Work out the finished part from the listing and answer in its coordinate system (mm). Give positions to 0.01 mm unless a question says otherwise; leave off trailing zeros. Write each loop counter-clockwise with the first axis right and the second up, starting at its lowest first coordinate (ties: lowest second). Pieces come first, ordered by that corner, then holes.
1) Given pin 1 Ø3 at (y, z) = (236, -1.5) entering from +X; pin 2 Ø5 at (y, z) = (98.5, 7.5) entering from +X; pin 3 Ø8 at (x, z) = (-358, -4) entering from -Y, each flat-ended and moving along its own axis, determine where each tip first touches the part or whether it passes through.
2) Straight lines are drawn through the part: probe 1 along X at (y, z) = (385.5, -10); probe 2 along X at (y, z) = (368, 12); probe 3 along Y at (x, z) = (-140.5, 21). For each, find the intervals that lie inside material, in ascending order.
3) Find section A-A (z = 8.5). Determine the outline of the cut face in (x, y) (1 decimal), plus the area to 3 significant figures.
4) Find section B-B (x = -89). Determine the outline of the cut face in (y, z), plus the area to 3 significant figures.
5) Find section C-C (y = 63). Determine the outline of the cut face in (x, z), plus the area to 3 significant figures.
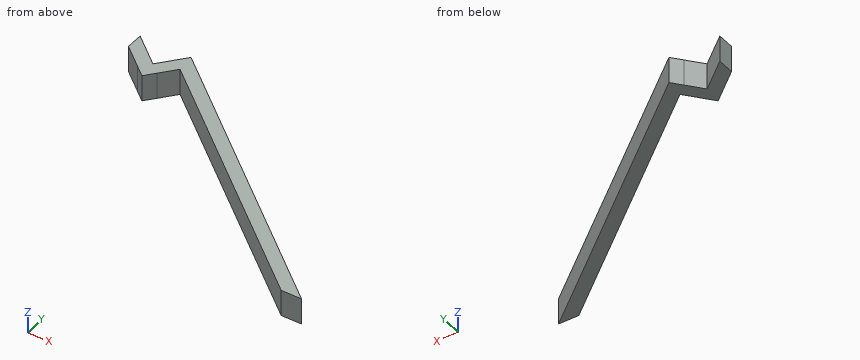
Autodesk Inventor part; units mm, degrees
ref_plane "YZ Plane" through (0, 0, 0) normal (1, 0, 0) x (0, 1, 0)
ref_plane "XZ Plane" through (0, 0, 0) normal (0, 1, 0) x (-1, 0, 0)
ref_plane "XY Plane" through (0, 0, 0) normal (0, 0, 1) x (1, 0, 0)
sketch "Sketch1" plane through (0, 0, 0) normal (0, 0, 1) x (1, 0, 0)
  line L0 (0, 0) -> (-505.8958, 424.4969)
  line L1 (0, 0) -> (-228.6, 0) construction
  line L2 (0, 0) -> (-39.5154, 0)
  line L3 (-39.5154, 0) -> (-502.765, 388.7126)
  line L4 (-505.8958, 424.4969) -> (-522.2226, 405.0394)
  line L5 (-522.2226, 405.0394) -> (-546.7128, 375.8531)
  line L6 (-527.2552, 359.5263) -> (-502.765, 388.7126)
  line L7 (-546.7128, 375.8531) -> (-605.0854, 424.8335)
  line L8 (-605.0854, 391.6762) -> (-563.0396, 356.3956)
  line L9 (-543.582, 340.0688) -> (-527.2552, 359.5263)
  line L10 (-563.0396, 356.3956) -> (-543.582, 340.0688)
  line L11 (-228.6, 0) -> (-203.2, 0)
  line L12 (-605.0854, 424.8335) -> (-605.0854, 391.6762)
  line L13 (0, 0) -> (0, 391.6762) construction
  dimension "d2" = 660.4
  dimension "d3" = 25.4
  dimension "d4" = 40
  dimension "d25" = 50
  dimension "d34" = 63.5
  dimension "d35" = 76.2
extrude "Extrusion1" add sketch "Sketch1" along normal mid plane 50.8
properties part number "newFrame1x2piecsV03"
Results:
1. pin 1: stops at x = -279.47
1. pin 2: stops at x = -114.41
1. pin 3: stops at y = 263.88
2. probe 1: x = -597.72 to -558.21, -538.62 to -505.46, -498.94 to -459.42
2. probe 2: x = -576.87 to -520.14, -478.08 to -438.57
2. probe 3: y = 84.74 to 117.89
3. outline: (-605.1, 391.7) - (-563, 356.4) - (-543.6, 340.1) - (-527.3, 359.5) - (-502.8, 388.7) - (-39.5, 0) - (0, 0) - (-505.9, 424.5) - (-522.2, 405) - (-546.7, 375.9) - (-605.1, 424.8) - close
3. area: 19,700 mm2
4. outline: (41.52, -25.4) - (74.68, -25.4) - (74.68, 25.4) - (41.52, 25.4) - close
4. area: 1,680 mm2
5. outline: (-114.6, -25.4) - (-75.08, -25.4) - (-75.08, 25.4) - (-114.6, 25.4) - close
5. area: 2,010 mm2
